Input: part model. Units: mm. Frame: model coordinates. Face numbers are marked on the shaded views. Give positions to 0.01 mm unless a question says otherwise; leave off trailing zeros. Loops run counter-clockwise (first coordinate to the right, second up) from the corner with the lowest first, then second, coordinate; pieces in that order, holes last. Notation, with made-up numbers: (87, 4.5) - (112, 4.5) arc R29 ccw to (112, 32.5) - close; hole circle Ø6 at (-31, -28). An arc over 180 degrees is marked (long way). Answer as a JSON object with one key per item and string values. Group by question number.
(1) Mould query, pull axis Z, two halves, no side actions, for the marked faces 1 and 2. Classes: +Z half, -Z half, draft (parallel to the pull), parting line (faces both ways), or undercut.
(2) Section query D-D (x = 25). Return loops of the section in (y, z), plus the area to 3 significant figures.
(3) Section query A-A (y = -1). Count the separate pieces of the cut face and the enclosed holes in it, plus the area to 3 significant figures.
(4) Material intervals for L1, parallel to X at y = -3, z = 0; L2, parallel to X at y = -0.85, z = 0; L3, parallel to Y at x = -17.5, z = 19, sorted ascending.
(5) Pin query (flat end, axial travel): P1, Ø0.8, axis at x = -24.5, z = 0, coming from the -Y side; P2, Ø3, axis at y = -2, z = -5, coming from the +X side; P3, Ø2, axis at x = -14, y = 1, coming from the +Z side. Return the tip coordinate at first contact, or that it passes through.
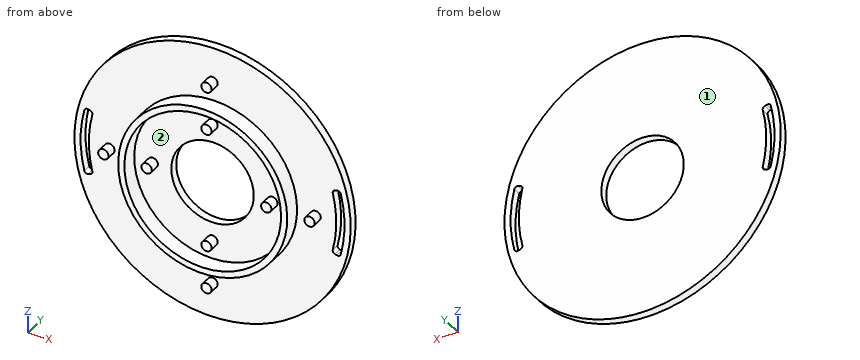
```python
from build123d import *

# Parameters (mm, degrees)
SKETCH_1_R          = 33.5
SKETCH_1_R_2        = 10
EXTRUDE_1_DEPTH     = 2
SKETCH_2_R          = 1.25
EXTRUDE_2_DEPTH     = 2.5
CUT_EXTRUDE_1_DEPTH = 2
SKETCH_4_R          = 20.5
SKETCH_4_R_2        = 19
EXTRUDE_3_DEPTH     = 4
SKETCH_5_R          = 1.25
EXTRUDE_4_DEPTH     = 2.5


with BuildPart() as part:
    # Эскиз1 → Бобышка-Вытянуть1 (new body)
    with BuildSketch(Plane(origin=(0, 0, 0), x_dir=(1, 0, 0), z_dir=(0, 1, 0))):
        with Locations(Location((0, 0, 0), (0, 0, 270))):
            Circle(SKETCH_1_R)
        with Locations(Location((0, 0, 0), (0, 0, 270))):
            Circle(SKETCH_1_R_2, mode=Mode.SUBTRACT)
    extrude(amount=EXTRUDE_1_DEPTH)

    # Эскиз2 → Бобышка-Вытянуть2 (add)
    with BuildSketch(Plane.XZ):
        with Locations(Location((0, 25, 0), (0, 0, 90))):
            Circle(SKETCH_2_R)
        with Locations(Location((-25, 0, 0), (0, 0, 90))):
            Circle(SKETCH_2_R)
        with Locations(Location((25, 0, 0), (0, 0, 90))):
            Circle(SKETCH_2_R)
        with Locations(Location((0, -25, 0), (0, 0, 90))):
            Circle(SKETCH_2_R)
    extrude(amount=EXTRUDE_2_DEPTH)

    # Эскиз3 → Вырез-Вытянуть1 (cut)
    with BuildSketch(Plane(origin=(0, 2, 0), x_dir=(1, 0, 0), z_dir=(0, 1, 0))):
        with BuildLine():
            Line((-29.693383157, 7.956318037), (-30.176487487, 8.085765453))
            ThreePointArc((-30.176487487, 8.085765453), (-30.753369556, 8.006293038), (-31.099496213, 7.537992789))
            ThreePointArc((-31.099496213, 7.537992789), (-32, 0), (-31.099496213, -7.537992789))
            ThreePointArc((-31.099496213, -7.537992789), (-30.753369556, -8.006293038), (-30.176487487, -8.085765453))
            Line((-30.176487487, -8.085765453), (-29.693383157, -7.956318037))
            ThreePointArc((-29.693383157, -7.956318037), (-29.242600206, -7.614767331), (-29.158534088, -7.055486505))
            ThreePointArc((-29.158534088, -7.055486505), (-30, 0), (-29.158534088, 7.055486505))
            ThreePointArc((-29.158534088, 7.055486505), (-29.242600206, 7.614767331), (-29.693383157, 7.956318037))
        make_face()
        with BuildLine():
            Line((29.693383157, -7.956318037), (30.176487487, -8.085765453))
            ThreePointArc((30.176487487, -8.085765453), (30.753369556, -8.006293038), (31.099496213, -7.537992789))
            ThreePointArc((31.099496213, -7.537992789), (32, 0), (31.099496213, 7.537992789))
            ThreePointArc((31.099496213, 7.537992789), (30.753369556, 8.006293038), (30.176487487, 8.085765453))
            Line((30.176487487, 8.085765453), (29.693383157, 7.956318037))
            ThreePointArc((29.693383157, 7.956318037), (29.242600206, 7.614767331), (29.158534088, 7.055486505))
            ThreePointArc((29.158534088, 7.055486505), (30, 0), (29.158534088, -7.055486505))
            ThreePointArc((29.158534088, -7.055486505), (29.242600206, -7.614767331), (29.693383157, -7.956318037))
        make_face()
    extrude(amount=-CUT_EXTRUDE_1_DEPTH, mode=Mode.SUBTRACT)

    # Эскиз4 → Бобышка-Вытянуть3 (add)
    with BuildSketch(Plane.XZ):
        with Locations(Location((0, 0, 0), (0, 0, 90))):
            Circle(SKETCH_4_R)
        with Locations(Location((0, 0, 0), (0, 0, 270))):
            Circle(SKETCH_4_R_2, mode=Mode.SUBTRACT)
    extrude(amount=EXTRUDE_3_DEPTH)

    # Эскиз5 → Бобышка-Вытянуть4 (add)
    with BuildSketch(Plane.XZ):
        with Locations(Location((0, 14.5, 0), (0, 0, 90))):
            Circle(SKETCH_5_R)
        with Locations(Location((14.5, 0, 0), (0, 0, 90))):
            Circle(SKETCH_5_R)
        with Locations(Location((0, -14.5, 0), (0, 0, 90))):
            Circle(SKETCH_5_R)
        with Locations(Location((-14.5, 0, 0), (0, 0, 90))):
            Circle(SKETCH_5_R)
    extrude(amount=EXTRUDE_4_DEPTH)


solid = part.part
```
Recorded:
{
 "1": {"face 1": "draft", "face 2": "undercut"},
 "2": {"outline": "(-2.5, -1.25) - (0, -1.25) - (0, -22.3) - (2, -22.3) - (2, 22.3) - (0, 22.3) - (0, 1.25) - (-2.5, 1.25) - close", "area": "95.4 mm^2"},
 "3": {"separate pieces": "9", "enclosed holes": "1", "area": "225 mm^2"},
 "4": {"L1": "x = -20.5 to -19, 19 to 20.5", "L2": "x = -26.25 to -23.75, -20.5 to -19, -15.75 to -13.25, 13.25 to 15.75, 19 to 20.5, 23.75 to 26.25", "L3": "y = 0 to 2"},
 "5": {"P1": "stops at y = -2.5", "P2": "stops at x = 20.2", "P3": "stops at z = 30.87"}
}
